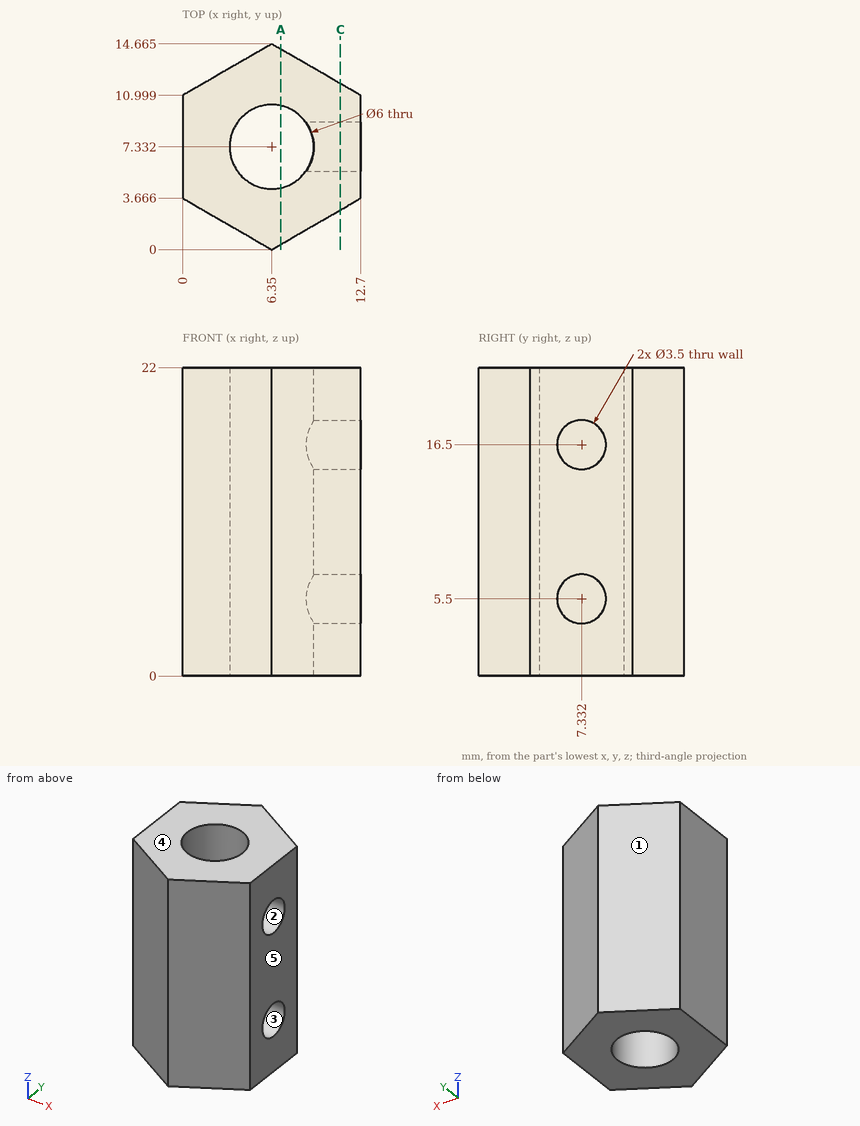
Verification items for this drawing (mm, ordinates from the low corner). A direction names the side the tool comes from. Round coordinates to 2 decimals unless told otherwise and drop trailing zeros. Order: outer loops, then holes, each group sorted by start corner. A loop starts at its lowest first (then second) coordinate and runs counter-clockwise, first axis right, second up. Notation, with made-up numbers: (-31.5, 69.25) - (-6.5, 69.25) arc R18 ccw to (-6.5, 99.25) - close; hole circle Ø4 at (46, 55.5). An arc over 180 degrees is marked (long way). Use CSV: the item, a comma, the result in double quotes. Start each with the question number.
1) Section check C-C, the plane x = 11.25. State how many separate pieces and enclosed holes the cut face has, plus the area to 3 significant figures.
2) Section check A-A, the plane x = 7. Record the cut outline in (y, z) (1 decimal), plus the area to 3 significant figures.
3) Access from +Z, -Z, +X, -X, +Y, -Y to the whole of each face (thin tool, end or side, straight path). Record for the marked faces 1 and 2.
4) Go/stop test with flat-tipped pins: P1, Ø1, axis at x = 7.5, z = 8.5, coming from the +Y side; P2, Ø3, axis at y = 7.33, z = 5.5, coming from the -X side; P3, Ø6, axis at x = 2.5, z = 10, coming from the +Y side (1 decimal); P4, Ø1.5, axis at x = 8, z = 8.5, coming from the -Y side. Record where each tip stops, or that it passes through.
5) Mould release check, pull along Z, two halves, no side actions. Record for the marked faces 3, 4 and 5: +Z half, -Z half, draft (parallel to the pull), parting line (faces both ways), or undercut.
6) Thickness scan on L1, parallel to Z at x = 12, y = 8.75 (1 decimal); L2, parallel to Y at x = 6.25, z = 14.5 (1 decimal); L3, parallel to Z at x = 10, y = 7.5. Record the ranges inside material, lowest first.
Answers:
1,separate pieces,"1"
1,enclosed holes,"2"
1,area,"179 mm²"
2,outline,"(0.4, 0) - (4.4, 0) - (4.4, 22) - (0.4, 22) - close; (10.3, 0) - (14.3, 0) - (14.3, 22) - (10.3, 22) - close"
2,area,"177 mm²"
3,face 1,"+Z, -Z, -X, +Y"
3,face 2,"+X"
4,P1,"stops at y = 14.29"
4,P2,"stops at x = 0"
4,P3,"stops at y = 14.2"
4,P4,"stops at y = 0.52"
5,face 3,"undercut"
5,face 4,"+Z half"
5,face 5,"draft"
6,L1,"z = 0 to 4.5, 6.5 to 15.5, 17.5 to 22"
6,L2,"y = 0.1 to 4.3, 10.3 to 14.6"
6,L3,"z = 0 to 3.76, 7.24 to 14.76, 18.24 to 22"
